Verification items for the finished model (mm, model axes). Face numbers are marked on the shaded views. Give positions to 0.01 mm unless a question says otherwise; leave off trailing zeros. Order: outer loops, then holes, each group sorted by start corner. A loop starts at its lowest first (then second) coordinate and runs counter-clockwise, first axis right, second up. Notation, with made-up numbers: (-0.75, 29.5) - (54.25, 29.5) arc R12 cw to (54.25, 37.5) - close; hole circle Ø7 at (54, 87.5). An arc over 180 degrees is marked (long way). Answer as a JSON object with one key per item and string values.
```python
from build123d import *

# Parameters (mm, degrees)
SKETCH1_R           = 23.8
BOSS_EXTRUDE1_DEPTH = 12
SKETCH2_W           = 268.538723742
SKETCH2_H           = 56.355455055
CUT_EXTRUDE1_DEPTH  = 26


with BuildPart() as part:
    # Sketch1 → Boss-Extrude1 (new body)
    with BuildSketch(Plane(origin=(0, 0, 0), x_dir=(1, 0, 0), z_dir=(0, 1, 0))):
        with BuildLine():
            Line((65, -39.8), (-65, -39.8))
            Line((-65, -39.8), (-96.605676951, -39.8))
            Line((-96.605676951, -39.8), (-96.605676951, -27.775552827))
            ThreePointArc((-96.605676951, -27.775552827), (-95.141210857, -24.240018922), (-91.605676951, -22.775552827))
            Line((-91.605676951, -22.775552827), (-69.589095412, -22.775552827))
            ThreePointArc((-69.589095412, -22.775552827), (-67.027094411, -22.069286735), (-65.188875184, -20.150013174))
            Line((-65.188875184, -20.150013174), (-42.066105387, 22.699840916))
            ThreePointArc((-42.066105387, 22.699840916), (0, 47.8), (42.066105387, 22.699840916))
            Line((42.066105387, 22.699840916), (65.188875184, -20.150013174))
            ThreePointArc((65.188875184, -20.150013174), (67.027094411, -22.069286735), (69.589095412, -22.775552827))
            Line((69.589095412, -22.775552827), (91.605676951, -22.775552827))
            ThreePointArc((91.605676951, -22.775552827), (95.141210857, -24.240018922), (96.605676951, -27.775552827))
            Line((96.605676951, -27.775552827), (96.605676951, -39.8))
            Line((96.605676951, -39.8), (65, -39.8))
        make_face()
        with Locations(Location((0, 0, 0), (0, 0, 270))):
            Circle(SKETCH1_R, mode=Mode.SUBTRACT)
    extrude(amount=BOSS_EXTRUDE1_DEPTH)

    # Sketch2 → Cut-Extrude1 (cut)
    with BuildSketch(Plane.XZ):
        with Locations((-8.696253547, 65.077727528)):
            Rectangle(SKETCH2_W, SKETCH2_H)
    extrude(amount=-CUT_EXTRUDE1_DEPTH, mode=Mode.SUBTRACT)


solid = part.part
```
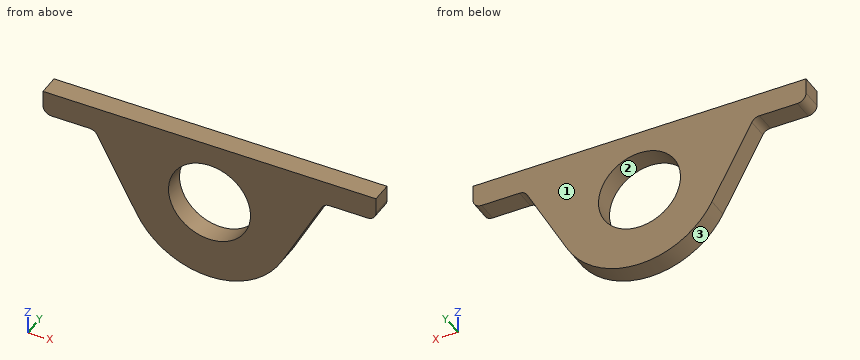
(1) Section check A-A (x = 0). Record the cut outline in (y, z).
Computed values:
{"outline": "(0, -47.8) - (12, -47.8) - (12, -23.8) - (0, -23.8) - close; (0, 23.8) - (12, 23.8) - (12, 36.9) - (0, 36.9) - close"}
(2) Section check D-D (x = 34). Record the cut outline in (y, z).
Computed values:
{"outline": "(0, -33.6) - (12, -33.6) - (12, 36.9) - (0, 36.9) - close"}
(3) Material ranges on line 1 along Z through (x, y) = (-1, 6); line 2 along Z through (x, y) = (79, 6.75); line 3 along X through (y, z) = (3.75, 11), recorded low to high. Write a range as [from, to].
Computed values:
{"line 1": "z = [-47.79, -23.78], [23.78, 36.9]", "line 2": "z = [22.78, 36.9]", "line 3": "x = [-60.25, -21.11], [21.11, 60.25]"}
(4) Release check for a two-part mould opening along X. For the marked faces 1, 2 and 3 record: pulls with the +X half, pulls with the -X half, needs draft (parallel to the pull), parting line crosses it, or undercut.
Computed values:
{"face 1": "needs draft", "face 2": "undercut", "face 3": "parting line crosses it"}
(5) Section check C-C (z = 10). Record the cut outline in (x, y), then the cut area to 3 significant figures.
Computed values:
{"outline": "(-59.71, 0) - (-21.6, 0) - (-21.6, 12) - (-59.71, 12) - close; (21.6, 0) - (59.71, 0) - (59.71, 12) - (21.6, 12) - close", "area": "915 mm²"}
(6) Gauge pin test, flat ends, axial feed: pin 1 Ø6 at (y, z) = (4, 24) entering from +X; pin 2 Ø1 at (y, z) = (4, 15) entering from -X; pin 3 Ø6 at (x, y) = (-31.5, 7.5) entering from -Z. Record the tip position at first contact, or that the pin passes through.
Computed values:
{"pin 1": "stops at x = 96.55", "pin 2": "stops at x = -62.68", "pin 3": "stops at z = -38.37"}
(7) Section check B-B (y = 9.5). Record the cut outline in (x, z).
Computed values:
{"outline": "(-96.61, 27.78) arc R5 ccw to (-91.61, 22.78) - (-69.59, 22.78) arc R5 cw to (-65.19, 20.15) - (-42.07, -22.7) arc R47.8 ccw to (42.07, -22.7) - (65.19, 20.15) arc R5 cw to (69.59, 22.78) - (91.61, 22.78) arc R5 ccw to (96.61, 27.78) - (96.61, 36.9) - (-96.61, 36.9) - close; hole circle Ø47.6 at (0, 0)"}
